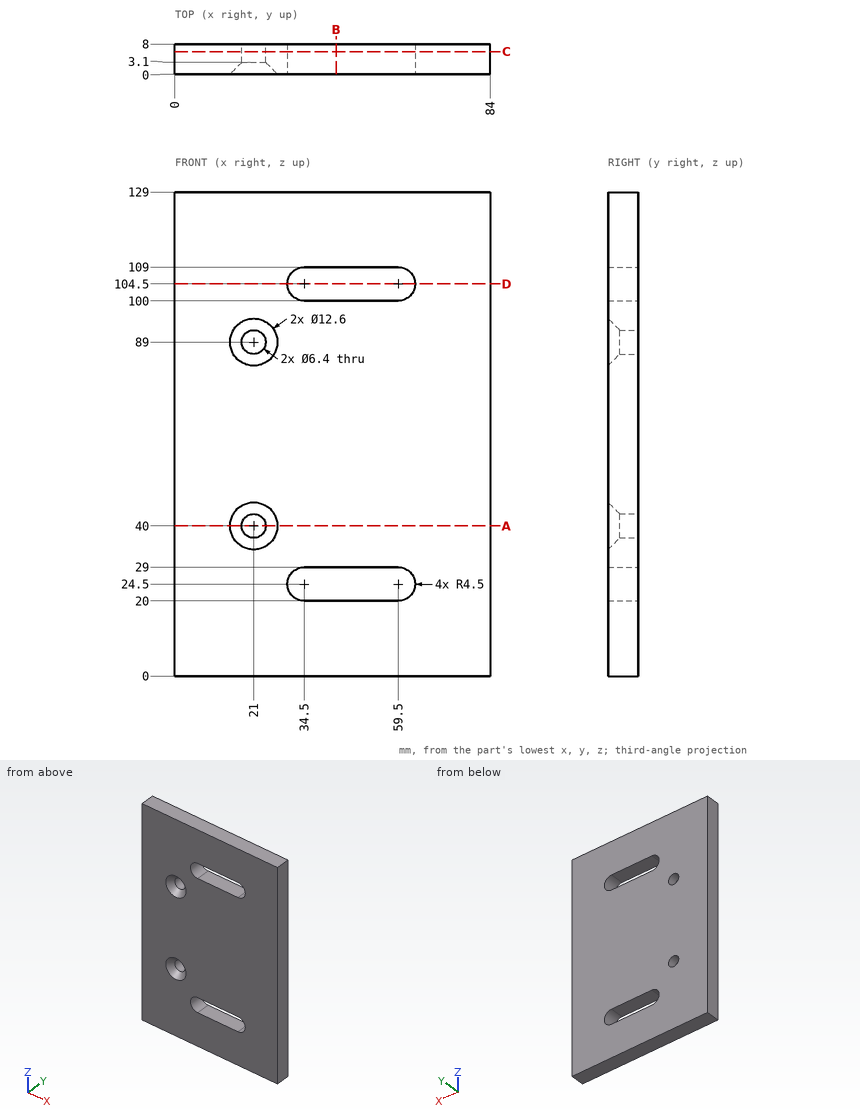
Geometry: see drawing. Coordinates: mm, zero at the bounding-box minimum. Give positions to 0.01 mm unless a question says otherwise; leave off trailing zeros. Order: outer loops, then holes, each group sorted by start corner. A loop starts at its lowest first (then second) coordinate and runs counter-clockwise, first axis right, second up.
Q1. Section B-B on x = 43. Output: boundary loops of the cut face in (y, z).
Checked values:
outline: (0, 0) - (8, 0) - (8, 20) - (0, 20) - close; (0, 29) - (8, 29) - (8, 100) - (0, 100) - close; (0, 109) - (8, 109) - (8, 129) - (0, 129) - close
Q2. Section D-D on z = 104.5. Output: boundary loops of the cut face in (x, y), and give its area (3 significant figures).
Checked values:
outline: (0, 0) - (30, 0) - (30, 8) - (0, 8) - close; (64, 0) - (84, 0) - (84, 8) - (64, 8) - close
area: 400 mm2
Q3. Ray query, probe 1 along Z at (x, y) = (21, 6.8); probe 2 along Z at (x, y) = (57, 7); probe 3 along X at (y, z) = (6.8, 89). Return the intervals inside material, ascending.
Checked values:
probe 1: z = 0 to 36.8, 43.2 to 85.8, 92.2 to 129
probe 2: z = 0 to 20, 29 to 100, 109 to 129
probe 3: x = 0 to 17.8, 24.2 to 84
Q4. Section A-A on z = 40. Output: boundary loops of the cut face in (x, y).
Checked values:
outline: (0, 0) - (14.7, 0) - (17.8, 3.1) - (17.8, 8) - (0, 8) - close; (24.2, 3.1) - (27.3, 0) - (84, 0) - (84, 8) - (24.2, 8) - close
Q5. Contact query for a flat-ended pin moving along its axis: pin 1 Ø1.5 at (y, z) = (2.5, 109) entering from -X. Output: stop coordinate, or through.
Checked values:
pin 1: stops at x = 0
Q6. Section C-C on y = 6. Output: boundary loops of the cut face in (x, z), and give its area (3 significant figures).
Checked values:
outline: (0, 0) - (84, 0) - (84, 129) - (0, 129) - close; hole circle Ø6.4 at (21, 40); hole circle Ø6.4 at (21, 89); hole (34.5, 20) - (59.5, 20) arc R4.5 ccw to (59.5, 29) - (34.5, 29) arc R4.5 ccw to start; hole (34.5, 100) - (59.5, 100) arc R4.5 ccw to (59.5, 109) - (34.5, 109) arc R4.5 ccw to start
area: 10,200 mm2
